from build123d import *

# Parameters (mm, degrees)
SKETCH2_R           = 1.35
BOSS_EXTRUDE1_DEPTH = 8.5
CUT_EXTRUDE1_DEPTH  = 6.4
CUT_EXTRUDE2_DEPTH  = 3.2


with BuildPart() as part:
    # Sketch2 → Boss-Extrude1 (new body, symmetric)
    with BuildSketch(Plane.XY):
        Circle(SKETCH2_R)
    extrude(amount=BOSS_EXTRUDE1_DEPTH, both=True)

    # Sketch4 → Cut-Extrude1 (cut)
    with BuildSketch(Plane(origin=(0, 0, -8.5), x_dir=(-1, 0, 0), z_dir=(0, 0, -1))):
        with BuildLine():
            Line((1, 0.906917857), (1, -0.906917857))
            ThreePointArc((1, -0.906917857), (1.35, 0), (1, 0.906917857))
        make_face()
    extrude(amount=-CUT_EXTRUDE1_DEPTH, mode=Mode.SUBTRACT)

    # Sketch5 → Cut-Extrude2 (cut)
    with BuildSketch(Plane.XY.offset(8.5)):
        with BuildLine():
            Line((-1, 0.906917857), (-1, -0.906917857))
            ThreePointArc((-1, -0.906917857), (-1.35, 0), (-1, 0.906917857))
        make_face()
    extrude(amount=-CUT_EXTRUDE2_DEPTH, mode=Mode.SUBTRACT)


solid = part.part
Can you work these out from the model? Positions are in its coordinate system, mm. A direction names the side the tool comes from. Round coordinates to 2 decimals unless told otherwise and drop trailing zeros. Order: outer loops, then holes, each group sorted by start corner. A loop starts at its lowest first (then second) coordinate and runs counter-clockwise, first axis right, second up. Notation, with made-up numbers: (-10, -9.5) - (6, -9.5) arc R17 ccw to (6, 4.5) - close; hole circle Ø6 at (-13, 51.5). An arc over 180 degrees is marked (long way). Answer in a Markdown table with one row per item.
(1) For P1, Ø0.9, axis at y = 0, z = 6.5, coming from the -X side, with a flat end and sliding along its axis, tell me the tip position at first contact or that it passes through.
From the geometry:
| item | result |
|---|---|
| P1 | stops at x = -1 |
(2) Which directions (+Z, -Z, +X, -X, +Y, -Y) give clear straight access to the entire face, cutting with the end or side of a thin tool? Please do faces 1 (the face through (0, 0, 8.5)), 2 (the face through (-1, 0, -5)), 3 (the face through (-1, 0, 7)).
From the geometry:
| item | result |
|---|---|
| face 1 | +Z, +X, -X, +Y, -Y |
| face 2 | -Z, -X, +Y, -Y |
| face 3 | +Z, -X, +Y, -Y |
(3) Suppose I cut it at A-A, the plane y = 0. Please give me the cut outline in (x, z), plus the area to 3 significant figures.
From the geometry:
| item | result |
|---|---|
| outline | (-1.35, -2.1) - (-1, -2.1) - (-1, -8.5) - (1.35, -8.5) - (1.35, 8.5) - (-1, 8.5) - (-1, 5.3) - (-1.35, 5.3) - close |
| area | 42.5 mm2 |
(4) Suppose I cut it at D-D, the plane y = -0.7. Please give me the cut outline in (x, z), plus the area to 3 significant figures.
From the geometry:
| item | result |
|---|---|
| outline | (-1.15, -2.1) - (-1, -2.1) - (-1, -8.5) - (1.15, -8.5) - (1.15, 8.5) - (-1, 8.5) - (-1, 5.3) - (-1.15, 5.3) - close |
| area | 37.8 mm2 |
(5) Suppose I cut it at C-C, the plane x = -0.25. Please give me the cut outline in (y, z).
From the geometry:
| item | result |
|---|---|
| outline | (-1.33, -8.5) - (1.33, -8.5) - (1.33, 8.5) - (-1.33, 8.5) - close |
(6) Suppose I cut it at B-B, the plane z = -1.25. Please give me the cut outline in (x, y), plus the area to 3 significant figures.
From the geometry:
| item | result |
|---|---|
| outline | circle Ø2.7 at (0, 0) |
| area | 5.73 mm2 |
(7) Please list where these lines run through material, in increasing order: L1, parallel to X at y = 0.05, z = -5.5; L2, parallel to Y at x = 0.2, z = -2.25; L3, parallel to Y at x = 0.95, z = 7.5. Write a range as from..to.
From the geometry:
| item | result |
|---|---|
| L1 | x = -1..1.35 |
| L2 | y = -1.34..1.34 |
| L3 | y = -0.96..0.96 |
